Here's how the part is built. I have some questions about the finished solid (model axes, mm). Face numbers are marked on the shaded views. A direction names the side the tool comes from. Round coordinates to 2 decimals unless told otherwise and drop trailing zeros. Loops run counter-clockwise (first coordinate to the right, second up) from the corner with the lowest first, then second, coordinate; pieces in that order, holes last. Notation, with made-up numbers: (68.25, 14.25) - (110.25, 14.25) arc R11 ccw to (110.25, 23.25) - close; hole circle Ø9 at (5, 87). An arc over 180 degrees is marked (long way). Answer as a JSON object with one key per item and string values. Group by question number.
1) Will these pins go through, and if not, where does the flat tip stop? P1, Ø1.5, axis at x = 0, z = 67.5, coming from the +Y side; P2, Ø4, axis at x = 8, z = 6, coming from the +Y side; P3, Ø5, axis at x = -8, z = 47.5, coming from the +Y side; P4, Ø5, axis at y = 35, z = -12.5, coming from the +X side.
2) Which directions (+Z, -Z, +X, -X, +Y, -Y) give clear straight access to the entire face, cutting with the end or side of a thin tool? Please do the marked faces 4, 5 and 6.
3) If we mould it in two halves opening along Z, with no side actions, what happens to the marked faces 1, 2 and 3? For each: pulls with the +Z half, pulls with the -Z half, needs draft (parallel to the pull), parting line crosses it, or undercut.
4) I want a section at A-A, the plane z = 64.5. Please give me the cut outline in (x, y).
5) I want a section at B-B, the plane y = -11. Please give me the cut outline in (x, z).
6) If I drill on line 1 along X through (y, z) = (0.4, -20.15) (3 decimals); line 2 along X through (y, z) = (24, 26) (3 decimals); line 3 along Z through (x, y) = (-6.5, 11), over which ranges is the centre line in solid material (lowest first)? Write a range as [from, to].
from build123d import *

# Parameters (mm, degrees)
BOSS_EXTRUDE2_DEPTH = 27
SKETCH5_R           = 3.8
BOSS_EXTRUDE3_DEPTH = 2
SKETCH6_R           = 2
CUT_EXTRUDE3_DEPTH  = 4
SKETCH7_R           = 9.25
BOSS_EXTRUDE4_DEPTH = 4.45
SKETCH8_R           = 4
BOSS_EXTRUDE5_DEPTH = 15.14
CUT_EXTRUDE4_START  = -13
CUT_EXTRUDE4_DEPTH  = 13
SKETCH11_R          = 15.5
BOSS_EXTRUDE6_DEPTH = 57
SKETCH12_R          = 6
BOSS_EXTRUDE7_DEPTH = 1.8
SKETCH13_R          = 1
BOSS_EXTRUDE8_DEPTH = 0.8
SKETCH14_R          = 1.25
CUT_EXTRUDE6_DEPTH  = 4
SKETCH10_R          = 2.05
CUT_EXTRUDE5_DEPTH  = 4


with BuildPart() as part:
    # Sketch1 → Boss-Extrude2 (new body)
    with BuildSketch(Plane(origin=(0, 0, 0), x_dir=(1, 0, 0), z_dir=(0, 1, 0))):
        with BuildLine():
            Line((17.005, -29), (-17.005, -29))
            ThreePointArc((-17.005, -29), (-19.126320344, -28.121320344), (-20.005, -26))
            Line((-20.005, -26), (-20.005, 26))
            ThreePointArc((-20.005, 26), (-19.126320344, 28.121320344), (-17.005, 29))
            Line((-17.005, 29), (17.005, 29))
            ThreePointArc((17.005, 29), (19.126320344, 28.121320344), (20.005, 26))
            Line((20.005, 26), (20.005, -26))
            ThreePointArc((20.005, -26), (19.126320344, -28.121320344), (17.005, -29))
        make_face()
    extrude(amount=BOSS_EXTRUDE2_DEPTH)

    # Sketch5 → Boss-Extrude3 (add)
    with BuildSketch(Plane(origin=(0, 27, 0), x_dir=(1, 0, 0), z_dir=(0, 1, 0))):
        with Locations(Location((-13.65, 20.15, 0), (0, 0, 90))):
            Circle(SKETCH5_R)
        with Locations(Location((13.65, 20.15, 0), (0, 0, 90))):
            Circle(SKETCH5_R)
        with Locations(Location((13.65, -20.2, 0), (0, 0, 90))):
            Circle(SKETCH5_R)
        with Locations(Location((-6.45, -6.7, 0), (0, 0, 90))):
            Circle(SKETCH5_R)
        with Locations(Location((6.45, -6.7, 0), (0, 0, 90))):
            Circle(SKETCH5_R)
        with BuildLine():
            Line((-16.798540367, -18.072397227), (-13.775104848, -13.598155653))
            ThreePointArc((-13.775104848, -13.598155653), (-8.498961708, -12.577218059), (-7.478024114, -17.853361199))
            Line((-7.478024114, -17.853361199), (-10.501459633, -22.327602773))
            ThreePointArc((-10.501459633, -22.327602773), (-15.777602773, -23.348540367), (-16.798540367, -18.072397227))
        make_face()
    boss_extrude3 = extrude(amount=BOSS_EXTRUDE3_DEPTH)

    # Sketch6 → Cut-Extrude3 (cut)
    with BuildSketch(Plane(origin=(0, 29, 0), x_dir=(1, 0, 0), z_dir=(0, 1, 0))):
        with Locations(Location((13.65, -20.2, 0), (0, 0, 270))):
            Circle(SKETCH6_R)
        with Locations(Location((13.65, 20.15, 0), (0, 0, 270))):
            Circle(SKETCH6_R)
        with Locations(Location((-13.65, 20.15, 0), (0, 0, 270))):
            Circle(SKETCH6_R)
        with Locations(Location((-13.65, -20.2, 0), (0, 0, 270))):
            Circle(SKETCH6_R)
    cut_extrude3 = extrude(amount=-CUT_EXTRUDE3_DEPTH, mode=Mode.SUBTRACT)

    # Sketch7 → Boss-Extrude4 (add)
    with BuildSketch(Plane(origin=(0, 27, 0), x_dir=(1, 0, 0), z_dir=(0, 1, 0))):
        with Locations(Location((0, 6, 0), (0, 0, 90))):
            Circle(SKETCH7_R)
    boss_extrude4 = extrude(amount=BOSS_EXTRUDE4_DEPTH)

    # Sketch8 → Boss-Extrude5 (add)
    with BuildSketch(Plane(origin=(0, 31.45, 0), x_dir=(1, 0, 0), z_dir=(0, 1, 0))):
        with Locations(Location((0, 6, 0), (0, 0, 270))):
            Circle(SKETCH8_R)
    boss_extrude5 = extrude(amount=BOSS_EXTRUDE5_DEPTH)

    # Sketch9 → Cut-Extrude4 (cut)
    with BuildSketch(Plane(origin=(0, 46.59, 0), x_dir=(1, 0, 0), z_dir=(0, 1, 0)).offset(CUT_EXTRUDE4_START)):
        with BuildLine():
            Line((-2.645751311, 9), (2.645751311, 9))
            ThreePointArc((2.645751311, 9), (0, 10), (-2.645751311, 9))
        make_face()
    cut_extrude4 = extrude(amount=CUT_EXTRUDE4_DEPTH, mode=Mode.SUBTRACT)

    # Mirror1: Boss-Extrude3, Cut-Extrude3, Boss-Extrude4, Boss-Extrude5, Cut-Extrude4 across plane
    add(boss_extrude3.mirror(Plane.ZX.offset(13.5)))
    add(cut_extrude3.mirror(Plane.ZX.offset(13.5)), mode=Mode.SUBTRACT)
    add(boss_extrude4.mirror(Plane.ZX.offset(13.5)))
    add(boss_extrude5.mirror(Plane.ZX.offset(13.5)))
    add(cut_extrude4.mirror(Plane.ZX.offset(13.5)), mode=Mode.SUBTRACT)

    # Sketch11 → Boss-Extrude6 (add)
    with BuildSketch(Plane.XY.offset(29)):
        with Locations(Location((0, 9.3, 0), (0, 0, 216.869897646))):
            Circle(SKETCH11_R)
    extrude(amount=BOSS_EXTRUDE6_DEPTH)

    # Sketch12 → Boss-Extrude7 (add)
    with BuildSketch(Plane.XY.offset(86)):
        with Locations((0, 9.3)):
            Circle(SKETCH12_R)
    extrude(amount=BOSS_EXTRUDE7_DEPTH)

    # Sketch13 → Boss-Extrude8 (add)
    with BuildSketch(Plane.XY.offset(87.8)):
        with Locations((0, 9.3)):
            Circle(SKETCH13_R)
    extrude(amount=BOSS_EXTRUDE8_DEPTH)

    # Sketch14 → Cut-Extrude6 (cut)
    with BuildSketch(Plane.XY.offset(86)):
        with Locations((9.854379173, 15.699508661)):
            Circle(SKETCH14_R)
        with Locations((-9.854379173, 2.900491339)):
            Circle(SKETCH14_R)
    extrude(amount=-CUT_EXTRUDE6_DEPTH, mode=Mode.SUBTRACT)

    # Sketch10 → Cut-Extrude5 (cut)
    with BuildSketch(Plane(origin=(0, 27, 0), x_dir=(1, 0, 0), z_dir=(0, 1, 0))):
        with Locations(Location((-17.6, 26.55, 0), (0, 0, 270))):
            Circle(SKETCH10_R)
        with Locations(Location((17.6, 26.55, 0), (0, 0, 270))):
            Circle(SKETCH10_R)
        with Locations(Location((17.6, -26.55, 0), (0, 0, 270))):
            Circle(SKETCH10_R)
        with Locations(Location((-17.6, -26.55, 0), (0, 0, 270))):
            Circle(SKETCH10_R)
    extrude(amount=-CUT_EXTRUDE5_DEPTH, mode=Mode.SUBTRACT)


solid = part.part
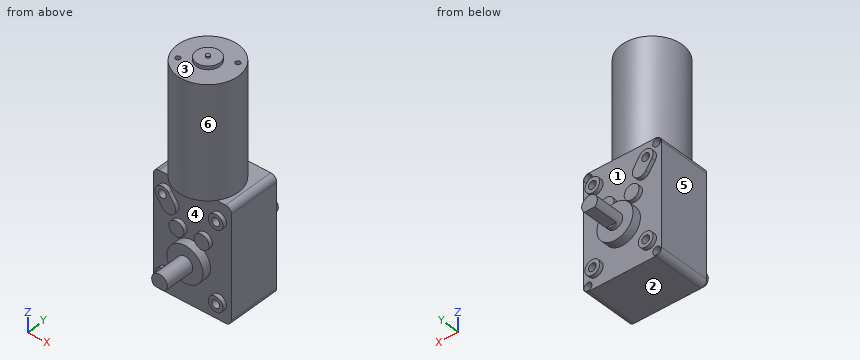
Outcome:
{
 "1": {"P1": "y = 24.8", "P2": "y = 29", "P3": "y = 23.79", "P4": "through"},
 "2": {"face 4": "-Y", "face 5": "+Z, -Z, -X, +Y, -Y", "face 6": "+Z"},
 "3": {"face 1": "undercut", "face 2": "pulls with the -Z half", "face 3": "pulls with the +Z half"},
 "4": {"outline": "circle Ø31 at (0, 9.3)"},
 "5": {"outline": "(-2.65, -9) - (2.65, -9) arc R4 ccw (long way) to start"},
 "6": {"line 1": "[-20.005, -15.65], [-11.65, 11.65], [15.65, 20.005]", "line 2": "[-20.005, -19.575], [-15.625, 15.625], [19.575, 20.005]", "line 3": "[-29, 86]"}
}
